Build history of the part. All positions in model axes, mm. Face numbers are marked on the shaded views. A direction names the side the tool comes from. Round coordinates to 2 decimals unless told otherwise and drop trailing zeros. Order: outer loops, then holes, each group sorted by start corner. A loop starts at its lowest first (then second) coordinate and runs counter-clockwise, first axis right, second up. Notation, with made-up numbers: (84, 64) - (103, 64) arc R32 ccw to (103, 100) - close; hole circle Ø9 at (16.5, 21). An arc over 180 degrees is marked (long way). Write each question's results on one line, items separated by ' | '. Start each with the question number.
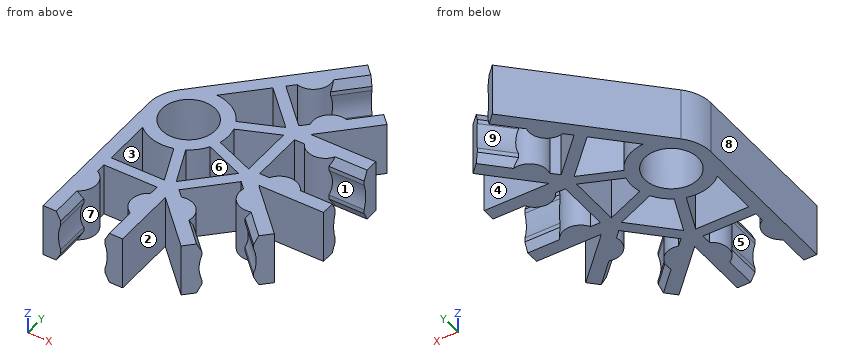
```python
from build123d import *

# Parameters (mm, degrees)
EXTRUDE_1_DEPTH          = 6
EXTRUDE_START            = -3.991967
EXTRUDE_2_DEPTH          = 3.991967
PATTERN_CIRCULAR_1_COUNT = 4
PATTERN_CIRCULAR_1_ANGLE = 135
SKETCH_4_R               = 3
CUT_EXTRUDE_1_DEPTH      = 7.0000001


with BuildPart() as part:
    # Sketch 1 → Extrude 1 (new body)
    with BuildSketch(Plane.XY):
        with BuildLine():
            Line((-4.5, 0), (-4.5, -18.2))
            Line((-4.5, -18.2), (-3, -18.2))
            Line((-3, -18.2), (-3, -14.6))
            ThreePointArc((-3, -14.6), (-1.968245837, -12.85), (-3, -11.1))
            Line((-3, -11.1), (-3, -10))
            Line((-3, -10), (3, -10))
            Line((3, -10), (3, -11.1))
            ThreePointArc((3, -11.1), (1.968245837, -12.85), (3, -14.6))
            Line((3, -14.6), (3, -18.2))
            Line((3, -18.2), (4.5, -18.2))
            Line((4.5, -18.2), (4.5, 0))
            ThreePointArc((4.5, 0), (0, 4.5), (-4.5, 0))
        make_face()
    extrude_1 = extrude(amount=EXTRUDE_1_DEPTH)

    # Sketch 3 → Extrude 2 (add)
    with BuildSketch(Plane.XZ.offset(18.2).offset(EXTRUDE_START)):
        with BuildLine():
            Line((-3, 6), (-3, 0))
            Line((-3, 0), (-2.5, 1))
            Line((-2.5, 1), (-2.5, 1.5))
            ThreePointArc((-2.5, 1.5), (-2.757359313, 3), (-2.5, 4.5))
            Line((-2.5, 4.5), (-2.5, 5))
            Line((-2.5, 5), (-3, 6))
        make_face()
        with BuildLine():
            Line((3, 0), (2.5, 1))
            Line((2.5, 1), (2.5, 1.5))
            ThreePointArc((2.5, 1.5), (2.757359313, 3), (2.5, 4.5))
            Line((2.5, 4.5), (2.5, 5))
            Line((2.5, 5), (3, 6))
            Line((3, 6), (3, 0))
        make_face()
    extrude_2 = extrude(amount=EXTRUDE_2_DEPTH)

    # Pattern Circular 1: Extrude 1, Extrude 2 ×4 about axis
    pattern_circular_1_axis = Axis((0, 0, 0), (0, 0, 1))
    for i in range(1, PATTERN_CIRCULAR_1_COUNT):
        add(extrude_1.rotate(pattern_circular_1_axis, i * PATTERN_CIRCULAR_1_ANGLE / (PATTERN_CIRCULAR_1_COUNT - 1)))
        add(extrude_2.rotate(pattern_circular_1_axis, i * PATTERN_CIRCULAR_1_ANGLE / (PATTERN_CIRCULAR_1_COUNT - 1)))

    # Sketch 4 → Cut-Extrude 1 (cut, through all)
    with BuildSketch(Plane(origin=(0, 0, 0), x_dir=(-1, 0, 0), z_dir=(0, 0, -1))):
        Circle(SKETCH_4_R)
        with BuildLine():
            Line((3, -8.75), (3, -3.354101966))
            ThreePointArc((3, -3.354101966), (1.038095674, -4.378625055), (-1.174936357, -4.343906601))
            Line((-1.174936357, -4.343906601), (-3, -8.75))
            Line((-3, -8.75), (3, -8.75))
        make_face()
        with BuildLine():
            Line((-8.308504679, -4.065863992), (-4.065863992, -8.308504679))
            Line((-4.065863992, -8.308504679), (-2.240800349, -3.90241128))
            ThreePointArc((-2.240800349, -3.90241128), (-3.181980515, -3.181980515), (-3.90241128, -2.240800349))
            Line((-3.90241128, -2.240800349), (-8.308504679, -4.065863992))
        make_face()
        with BuildLine():
            Line((-8.75, -3), (-4.343906601, -1.174936357))
            ThreePointArc((-4.343906601, -1.174936357), (-4.5, 0), (-4.343906601, 1.174936357))
            Line((-4.343906601, 1.174936357), (-8.75, 3))
            Line((-8.75, 3), (-8.75, -3))
        make_face()
        with BuildLine():
            Line((-4.065863992, 8.308504679), (-0.250387902, 4.493028589))
            ThreePointArc((-0.250387902, 4.493028589), (-2.362110978, 3.830199959), (-3.90241128, 2.240800349))
            Line((-3.90241128, 2.240800349), (-8.308504679, 4.065863992))
            Line((-8.308504679, 4.065863992), (-4.065863992, 8.308504679))
        make_face()
    extrude(amount=-CUT_EXTRUDE_1_DEPTH, mode=Mode.SUBTRACT)


solid = part.part
```
1. Cut at B-B (x = 13). Give the number of separate pieces and of enclosed holes in the cut face, plus the area to 3 significant figures.
2. Wall check: line 1 (Y direction, x = 0, z = 1.9); line 2 (X direction, y = -5.5, z = 0.5); line 3 (X direction, y = -4, z = 2.25). Give the ranges that are in metal, low to high. Write a range as from..to.
3. Cut at A-A (x = 16.5). List the corners of the cut face in (y, z).
4. 3-axis set-ups, long thin cutter, end or side, ignore diameter. For the marked faces 1, 2, 3, 4 and 5: which of +Z, -Z, +X, -X, +Y, -Y reach the whole face in a straight line?
5. Mould opens along Y. For the marked faces 6, 7, 8 and 9 say: pulls with the +Y half, pulls with the -Y half, needs draft (parallel to the pull), parting line crosses it, or undercut.
6. Flat gauge pins, fed straight in: pin 1 Ø2 at (x, z) = (13.5, 5) entering from +Y; pin 2 Ø12 at (x, y) = (0.5, -13.5) entering from -Z; pin 3 Ø1.5 at (y, z) = (-8.5, 3.5) entering from +X; pin 4 Ø3 at (x, z) = (14, 3.5) entering from +Y. Where does each tip first touch, or does it go through?
A:
1) separate pieces: 4 | enclosed holes: 0 | area: 61.4 mm^2
2) line 1: y = -10..-8.75, -4.5..-3, 3..6.36 | line 2: x = -4.5..-3, 1.65..2.9, 6.87..8.64, 9.74..11.86 | line 3: x = -4.5..-3, -2.06..2.28, 8.15..18.2
3) outline: (-4.5, 0) - (-3, 0) - (-2.5, 1) - (-2.5, 1.5) arc R4.5 cw to (-2.5, 4.5) - (-2.5, 5) - (-3, 6) - (-4.5, 6) - close; (2.5, 1) - (3, 0) - (4.5, 0) - (4.5, 6) - (3, 6) - (2.5, 5) - (2.5, 4.5) arc R4.5 cw to (2.5, 1.5) - close
4) face 1: +X | face 2: +Z, -Z, -Y | face 3: +Z, -Z | face 4: +Z, -Z, +X | face 5: -Y
5) face 6: undercut | face 7: undercut | face 8: needs draft | face 9: pulls with the +Y half
6) pin 1: stops at y = 10.96 | pin 2: stops at z = 0 | pin 3: stops at x = 15.61 | pin 4: stops at y = 11.1
